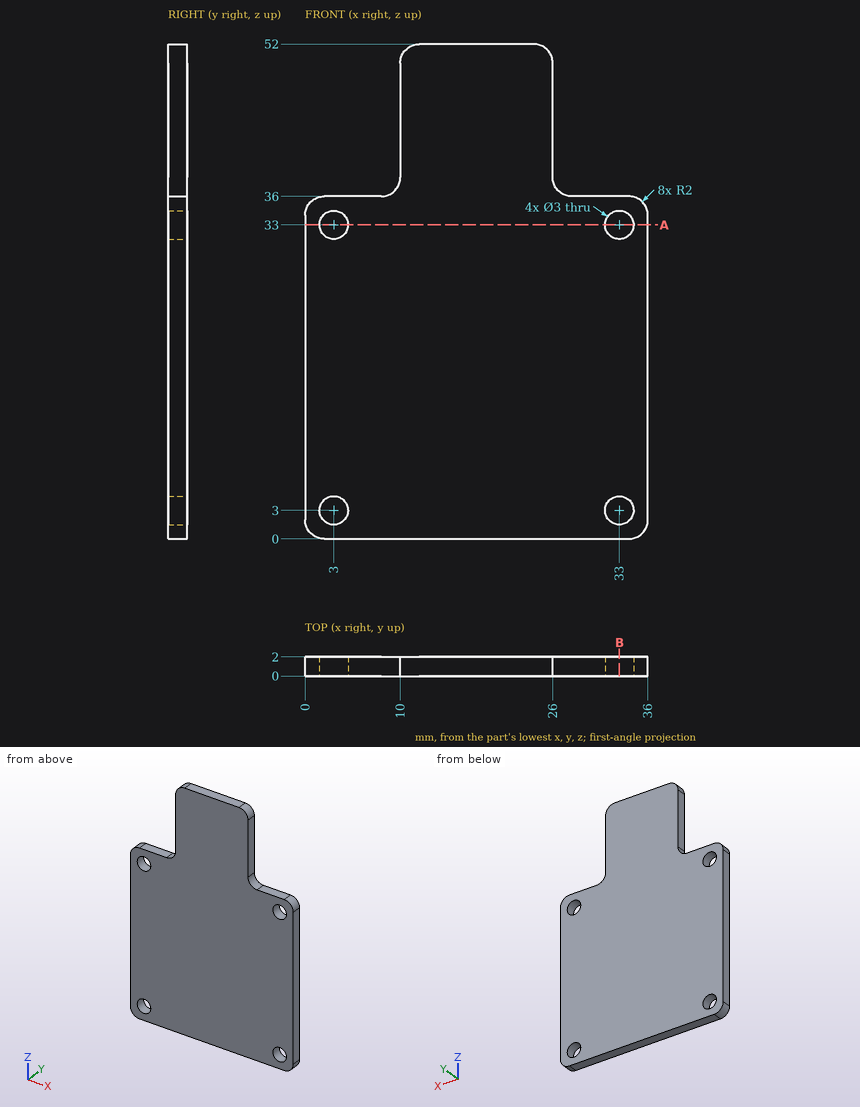
Answer from the drawing. Dimensions are ordinates in mm from the lowest x, y and z of the part. Coordinates: 2 decimals unless noted, no trailing zeros. Loops run counter-clockwise (first coordinate to the right, second up) from the corner with the lowest first, then second, coordinate; pieces in that order, holes last.
1) Section A-A (z = 33) is taken. Give the vertices of the cut face in (x, y), plus the area to 3 significant figures.
Results:
outline: (0, 0) - (1.5, 0) - (1.5, 2) - (0, 2) - close; (4.5, 0) - (31.5, 0) - (31.5, 2) - (4.5, 2) - close; (34.5, 0) - (36, 0) - (36, 2) - (34.5, 2) - close
area: 60.0 mm2
2) Flat-ended cylindrical pins translate along their axes: pin 1 (2.5 mm diameter, centred on x = 33, z = 33, fed in from -Y); pin 2 (5 mm diameter, centred on x = 7.5, z = 26.5, fed in from -Y); pin 3 (1 mm diameter, centred on y = 1, z = 38, fed in from +X); pin 4 (1 mm diameter, centred on y = 1, z = 44.5, fed in from +X). Find the tip coordinate at first contact, or state that the pin passes through.
Results:
pin 1: passes through
pin 2: stops at y = 0
pin 3: stops at x = 26.06
pin 4: stops at x = 26
3) Consider probe 1 along X at (y, z) = (0.7, 33); probe 2 along X at (y, z) = (1.5, 32.5); probe 3 along X at (y, z) = (1.4, 41). Determine where each line is inside the solid, lowest interval first.
Results:
probe 1: x = 0 to 1.5, 4.5 to 31.5, 34.5 to 36
probe 2: x = 0 to 1.59, 4.41 to 31.59, 34.41 to 36
probe 3: x = 10 to 26
4) Section B-B (x = 33) is taken. Give the vertices of the cut face in (y, z).
Results:
outline: (0, 0) - (2, 0) - (2, 1.5) - (0, 1.5) - close; (0, 4.5) - (2, 4.5) - (2, 31.5) - (0, 31.5) - close; (0, 34.5) - (2, 34.5) - (2, 36) - (0, 36) - close
